Check sheet for the modelled part. Datum: model origin and axes. Units: mm. Face numbers are marked on the shaded views. Round coordinates to 2 decimals unless told otherwise and drop trailing zeros. Write each loop counter-clockwise with the first axis right and the second up, starting at its lowest first coordinate (ties: lowest second). Pieces come first, ordered by that corner, then holes. Notation, with made-up numbers: (3.5, 48.25) -> (39.5, 48.25) arc R30 cw to (39.5, 78.25) -> close; hole circle Ø8 at (65, 76.25). An arc over 180 degrees is marked (long way). Answer as a JSON object with one key per item and string values. Group by question number.
```python
from build123d import *

# Parameters (mm, degrees)
SKETCH1_R                 = 1.651
BOSS_EXTRUDE2_DEPTH       = 6.35
SKETCH2_R                 = 1.143
CUT_EXTRUDE1_DEPTH        = 7.35
SKETCH3_R                 = 12.1285
CUT_EXTRUDE2_DEPTH        = 7.35
SKETCH4_W                 = 28.562713242
SKETCH4_H                 = 11.677503754
BOSS_EXTRUDE3_DEPTH       = 6.35
SKETCH5_W                 = 216.7214489
SKETCH5_H                 = 130.569220634
CUT_EXTRUDE4_DEPTH        = 7.35
SKETCH6_R                 = 38.1
CUT_EXTRUDE5_DEPTH        = 60.96
FILLET1_R                 = 6.35
FILLET2_R                 = 6.35
SKETCH102_W               = 8.89
SKETCH102_H               = 8.89
CUT_EXTRUDE101_DEPTH      = 7.3500001
SKETCH105_R               = 5
CUT_EXTRUDE104_DEPTH      = 10
SKETCH106_R               = 3.175
CUT_EXTRUDE105_DEPTH      = 103.378
CUT_EXTRUDE105_DEPTH_BACK = 1
SKETCH158_R               = 1.651
CUT_EXTRUDE157_DEPTH      = 97.79


with BuildPart() as part:
    # Sketch1 → Boss-Extrude2 (new body)
    with BuildSketch(Plane.XY):
        with BuildLine():
            Line((-64.964441474, 37.338), (-54.550441474, 37.338))
            Line((-54.550441474, 37.338), (-54.550441474, -37.338))
            Line((-54.550441474, -37.338), (-64.964441474, -37.338))
            ThreePointArc((-64.964441474, -37.338), (0, -74.93), (64.964441474, -37.338))
            Line((64.964441474, -37.338), (54.550441474, -37.338))
            Line((54.550441474, -37.338), (54.550441474, 37.338))
            Line((54.550441474, 37.338), (64.964441474, 37.338))
            ThreePointArc((64.964441474, 37.338), (0, 74.93), (-64.964441474, 37.338))
        make_face()
        with Locations((-46.482, 11.049)):
            Circle(SKETCH1_R, mode=Mode.SUBTRACT)
        with Locations((-21.083270032, 10.795)):
            Circle(SKETCH1_R, mode=Mode.SUBTRACT)
        with Locations((-21.083270032, -10.795)):
            Circle(SKETCH1_R, mode=Mode.SUBTRACT)
        with Locations((-46.482, -11.049)):
            Circle(SKETCH1_R, mode=Mode.SUBTRACT)
        with Locations((46.482, -11.049)):
            Circle(SKETCH1_R, mode=Mode.SUBTRACT)
        with Locations((21.083270032, -10.795)):
            Circle(SKETCH1_R, mode=Mode.SUBTRACT)
        with Locations((21.083270032, 10.795)):
            Circle(SKETCH1_R, mode=Mode.SUBTRACT)
        with Locations((46.482, 11.049)):
            Circle(SKETCH1_R, mode=Mode.SUBTRACT)
    extrude(amount=BOSS_EXTRUDE2_DEPTH)

    # Sketch2 → Cut-Extrude1 (cut, through all)
    with BuildSketch(Plane.XY.offset(6.35)):
        with Locations((-6.731, 62.23)):
            Circle(SKETCH2_R)
        with Locations((6.731, 62.23)):
            Circle(SKETCH2_R)
    extrude(amount=-CUT_EXTRUDE1_DEPTH, mode=Mode.SUBTRACT)

    # Sketch3 → Cut-Extrude2 (cut, through all)
    with BuildSketch(Plane(origin=(0, 0, 0), x_dir=(-1, 0, 0), z_dir=(0, 0, -1))):
        with Locations((-43.105229381, -43.105229381)):
            Circle(SKETCH3_R)
        with Locations((14.224, -34.29)):
            Circle(SKETCH3_R)
        with Locations((14.224, 34.29)):
            Circle(SKETCH3_R)
        with Locations((-43.105229381, 43.105229381)):
            Circle(SKETCH3_R)
        with Locations((43.105229381, 43.105229381)):
            Circle(SKETCH3_R)
        with Locations((-14.224, 34.29)):
            Circle(SKETCH3_R)
        with Locations((-14.224, -34.29)):
            Circle(SKETCH3_R)
        with Locations((43.105229381, -43.105229381)):
            Circle(SKETCH3_R)
    extrude(amount=-CUT_EXTRUDE2_DEPTH, mode=Mode.SUBTRACT)

    # Sketch4 → Boss-Extrude3 (add)
    with BuildSketch(Plane(origin=(0, 0, 0), x_dir=(-1, 0, 0), z_dir=(0, 0, -1))):
        with Locations((-1.488809975, 62.152540216)):
            Rectangle(SKETCH4_W, SKETCH4_H)
    extrude(amount=-BOSS_EXTRUDE3_DEPTH)

    # Sketch5 → Cut-Extrude4 (cut, through all)
    with BuildSketch(Plane(origin=(0, 0, 0), x_dir=(-1, 0, 0), z_dir=(0, 0, -1))):
        with Locations((23.316688373, 48.139610317)):
            Rectangle(SKETCH5_W, SKETCH5_H)
    extrude(amount=-CUT_EXTRUDE4_DEPTH, mode=Mode.SUBTRACT)

    # Sketch6 → Cut-Extrude5 (cut)
    with BuildSketch(Plane(origin=(0, 0, 0), x_dir=(-1, 0, 0), z_dir=(0, 0, -1))):
        with Locations((0, -86.312058398)):
            Circle(SKETCH6_R)
    extrude(amount=-CUT_EXTRUDE5_DEPTH, mode=Mode.SUBTRACT)

    # Fillet1
    fillet1_edges = [part.edges().sort_by_distance(p)[0] for p in [
        (-33.000960548, -67.271401821, 3.175),
    ]]
    fillet(fillet1_edges, radius=FILLET1_R)

    # Fillet2
    fillet2_edges = [part.edges().sort_by_distance(p)[0] for p in [
        (33.000960548, -67.271401821, 3.175),
    ]]
    fillet(fillet2_edges, radius=FILLET2_R)

    # Sketch102 → Cut-Extrude101 (cut, through all)
    with BuildSketch(Plane(origin=(0, 0, 0), x_dir=(-1, 0, 0), z_dir=(0, 0, -1))):
        with Locations((-33.605441474, -21.59)):
            Rectangle(SKETCH102_W, SKETCH102_H)
        with Locations((33.605441474, -21.59)):
            Rectangle(SKETCH102_W, SKETCH102_H)
    extrude(amount=-CUT_EXTRUDE101_DEPTH, mode=Mode.SUBTRACT)

    # Sketch105 → Cut-Extrude104 (cut)
    with BuildSketch(Plane(origin=(0, 0, 0), x_dir=(-1, 0, 0), z_dir=(0, 0, -1))):
        with Locations((-12.7, -15.24)):
            Circle(SKETCH105_R)
        with Locations((12.7, -15.24)):
            Circle(SKETCH105_R)
    extrude(amount=-CUT_EXTRUDE104_DEPTH, mode=Mode.SUBTRACT)

    # Sketch106 → Cut-Extrude105 (cut, two sides)
    with BuildSketch(Plane(origin=(30.092005081, 4.08352975, 25.4), x_dir=(-1, 0, 0), z_dir=(0, 0, -1))) as cut_extrude105_sk:
        with Locations((73.272005081, -29.48352975)):
            Circle(SKETCH106_R)
        with Locations((30.092005081, -29.48352975)):
            Circle(SKETCH106_R)
        with Locations((-13.087994919, -29.48352975)):
            Circle(SKETCH106_R)
    extrude(amount=CUT_EXTRUDE105_DEPTH, mode=Mode.SUBTRACT)
    extrude(cut_extrude105_sk.sketch, amount=-CUT_EXTRUDE105_DEPTH_BACK, mode=Mode.SUBTRACT)

    # Sketch158 → Cut-Extrude157 (cut)
    with BuildSketch(Plane(origin=(30.092005081, 4.08352975, -22.225), x_dir=(-1, 0, 0), z_dir=(0, 0, -1))):
        with Locations((4.154396091, -49.728759131)):
            Circle(SKETCH158_R)
        with Locations((56.02961407, -49.728759131)):
            Circle(SKETCH158_R)
    extrude(amount=-CUT_EXTRUDE157_DEPTH, mode=Mode.SUBTRACT)


solid = part.part
```
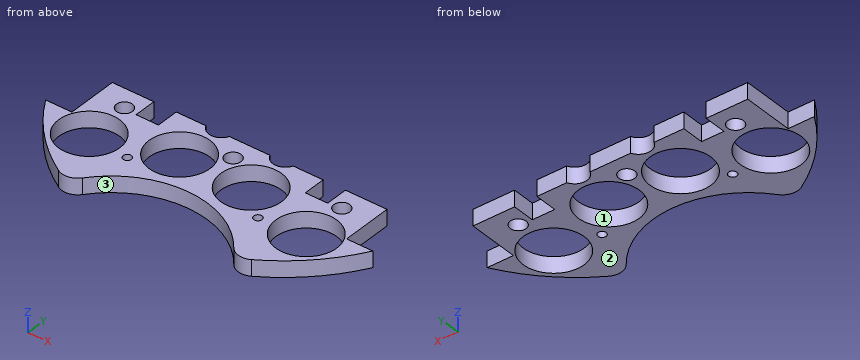
(1) Scan lines: line 1 along X through (y, z) = (-27, 0.75); line 2 along X through (y, z) = (-42.5, 4.75); line 3 along X through (y, z) = (-43, 1). Record each from-to range of solid material in increasing order.
(2) Section check D-D on y = -34.29. Record the cut outline in (x, z), then the cut area to 3 significant figures.
(3) Section check B-B on y = -24. State how many separate pieces and enclosed holes the cut face has, then the cut area to 3 significant figures.
(4) Go/stop test with flat-tipped pins: pin 1 Ø3 at (y, z) = (-23, 4) entering from +X; pin 2 Ø3 at (x, z) = (-34, 2.5) entering from +Y (3 decimals); pin 3 Ø2 at (x, y) = (46, -60) entering from +Z; pin 4 Ø1.9 at (x, z) = (-58.5, 3) entering from +Y. Record where each tip stops, or that it passes through.
(5) Section check A-A on x = 0. Record the cut outline in (y, z) (3 decimals).
(6) Release check for a two-part mould opening along Y. For the marked faces 1, 2 and 3 record: pulls with the +Y half, pulls with the -Y half, needs draft (parallel to the pull), parting line crosses it, or undercut.
Data:
{
 "1": {"line 1": "x = -54.55 to -45.92, -40.44 to -23.92, -4.53 to -2.74, 2.74 to 4.53, 23.92 to 40.44, 45.92 to 54.55", "line 2": "x = -61.71 to -55.22, -30.99 to -23.15, -5.3 to 5.3, 23.15 to 30.99, 55.22 to 61.71", "line 3": "x = -61.36 to -55.23, -30.98 to -22.66, -5.78 to 5.78, 22.66 to 30.98, 55.23 to 61.36"},
 "2": {"outline": "(-54.55, 0) -> (-51.44, 0) -> (-51.44, 6.35) -> (-54.55, 6.35) -> close; (-34.78, 0) -> (-26.35, 0) -> (-26.35, 6.35) -> (-34.78, 6.35) -> close; (-2.1, 0) -> (2.1, 0) -> (2.1, 6.35) -> (-2.1, 6.35) -> close; (26.35, 0) -> (34.78, 0) -> (34.78, 6.35) -> (26.35, 6.35) -> close; (51.44, 0) -> (54.55, 0) -> (54.55, 6.35) -> (51.44, 6.35) -> close", "area": "173 mm²"},
 "3": {"separate pieces": "8", "enclosed holes": "0", "area": "308 mm²"},
 "4": {"pin 1": "stops at x = 54.55", "pin 2": "stops at y = -26.035", "pin 3": "stops at z = 6.35", "pin 4": "stops at y = -37.34"},
 "5": {"outline": "(-48.212, 0) -> (-28.575, 0) -> (-28.575, 6.35) -> (-48.212, 6.35) -> close; (-22.225, 0) -> (-17.145, 0) -> (-17.145, 6.35) -> (-22.225, 6.35) -> close"},
 "6": {"face 1": "undercut", "face 2": "needs draft", "face 3": "pulls with the -Y half"}
}
